Could you check a few things on this model? Use its own coordinates, in mm. A direction names the side the tool comes from. Coordinates: 2 decimals unless noted, no trailing zeros. Loops run counter-clockwise (first coordinate to the right, second up) from the corner with the lowest first, then second, coordinate; pieces in that order, holes last. Notation, with made-up numbers: (24.5, -39) - (52.5, -39) arc R27 ccw to (52.5, -21) - close; hole circle Ø5 at (-20, -38.5). An arc over 180 degrees is marked (long way). Use CSV: the item, a comma, the result in double quotes.
from build123d import *

# Parameters (mm, degrees)
SKETCH1_R               = 27.5
BOSS_EXTRUDE1_DEPTH     = 8
SKETCH2_R               = 26.25
BOSS_EXTRUDE2_DEPTH     = 11
BOSS_EXTRUDE3_DEPTH     = 8
SKETCH4_R               = 5
CUT_EXTRUDE1_DEPTH      = 54.872534746
MIRROR2_OUTLINE_R       = 5
MIRROR2_DEPTH           = 8
SKETCH6_R               = 15
BOSS_EXTRUDE4_DEPTH     = 7
CUT_EXTRUDE2_DEPTH      = 57.055775795
CUT_EXTRUDE2_DEPTH_BACK = 57.055775795
SKETCH5_R               = 10


# Read off the part's stored shape, not the designer's step: Mirror2
with BuildPart() as part:
    # Sketch1 → Boss-Extrude1 (new body)
    with BuildSketch(Plane(origin=(0, 0, 0), x_dir=(1, 0, 0), z_dir=(0, 1, 0))):
        with Locations(Location((0, 0, 0), (0, 0, 270))):
            Circle(SKETCH1_R)
    extrude(amount=BOSS_EXTRUDE1_DEPTH)

    # Sketch2 → Boss-Extrude2 (add)
    with BuildSketch(Plane(origin=(0, 8, 0), x_dir=(1, 0, 0), z_dir=(0, 1, 0))):
        with Locations(Location((0, 0, 0), (0, 0, 270))):
            Circle(SKETCH2_R)
    extrude(amount=BOSS_EXTRUDE2_DEPTH)

    # Sketch3 → Boss-Extrude3 (add)
    with BuildSketch(Plane(origin=(0, 0, 0), x_dir=(1, 0, 0), z_dir=(0, 1, 0))):
        Polygon((20.794342335, 16.0205439), (44.474731406, 6.832149094), (45, 0), (20.794342335, 0), align=None)
    boss_extrude3 = extrude(amount=BOSS_EXTRUDE3_DEPTH)

    # Mirror1: Boss-Extrude3 across plane
    add(boss_extrude3.mirror(Plane.XY))

    # Sketch4 → Cut-Extrude1 (cut, through all)
    with BuildSketch(Plane(origin=(0, 8, 0), x_dir=(1, 0, 0), z_dir=(0, 1, 0))):
        with Locations(Location((35.5, 0, 0), (0, 0, 270))):
            Circle(SKETCH4_R)
    extrude(amount=-CUT_EXTRUDE1_DEPTH, mode=Mode.SUBTRACT)

    # Mirror2 outline → Mirror2 (add)
    with BuildSketch(Plane(origin=(0, 0, 0), x_dir=(1, 0, 0), z_dir=(0, 1, 0))):
        with BuildLine():
            ThreePointArc((-22.9203732, -15.195607667), (-27.5, 0), (-22.9203732, 15.195607667))
            Line((-22.9203732, 15.195607667), (-44.474731406, 6.832149094))
            Line((-44.474731406, 6.832149094), (-45, 0))
            Line((-45, 0), (-44.474731406, -6.832149094))
            Line((-44.474731406, -6.832149094), (-22.9203732, -15.195607667))
        make_face()
        with Locations((-35.5, 0)):
            Circle(MIRROR2_OUTLINE_R, mode=Mode.SUBTRACT)
    extrude(amount=MIRROR2_DEPTH)

    # Sketch6 → Boss-Extrude4 (add)
    with BuildSketch(Plane(origin=(0, 19, 0), x_dir=(1, 0, 0), z_dir=(0, 1, 0))):
        with Locations(Location((0, 0, 0), (0, 0, 270))):
            Circle(SKETCH6_R)
    extrude(amount=BOSS_EXTRUDE4_DEPTH)

    # Sketch5 → Cut-Extrude2 (cut, two sides: drawn at the far end of the back side and taken through both)
    with BuildSketch(Plane(origin=(0, 19, 0), x_dir=(1, 0, 0), z_dir=(0, 1, 0)).offset(-CUT_EXTRUDE2_DEPTH_BACK)):
        with Locations(Location((0, 0, 0), (0, 0, 270))):
            Circle(SKETCH5_R)
    extrude(amount=CUT_EXTRUDE2_DEPTH + CUT_EXTRUDE2_DEPTH_BACK, mode=Mode.SUBTRACT)


solid = part.part
(1) Suppose I cut it at B-B (y = 2.5). Write out the boundary of the cut face in (x, z), plus the area to 3 significant figures.
Computed:
outline,"(-45, 0) - (-44.47, -6.83) - (-22.92, -15.2) arc R27.5 ccw to (22.92, -15.2) - (44.47, -6.83) - (45, 0) - (44.47, 6.83) - (22.92, 15.2) arc R27.5 ccw to (-22.92, 15.2) - (-44.47, 6.83) - close; hole circle Ø10 at (-35.5, 0); hole circle Ø20 at (0, 0); hole circle Ø10 at (35.5, 0)"
area,"2,670 mm²"
(2) Suppose I cut it at A-A (x = 0). Write out the boundary of the cut face in (y, z), plus the area to 4 significant figures.
Computed:
outline,"(0, -27.5) - (8, -27.5) - (8, -26.25) - (19, -26.25) - (19, -15) - (26, -15) - (26, -10) - (0, -10) - close; (0, 10) - (26, 10) - (26, 15) - (19, 15) - (19, 26.25) - (8, 26.25) - (8, 27.5) - (0, 27.5) - close"
area,"707.5 mm²"
(3) Suppose I cut it at D-D (y = 16.75). Write out the boundary of the cut face in (x, z).
Computed:
outline,"circle Ø52.5 at (0, 0); hole circle Ø20 at (0, 0)"
(4) Will these pins go through, and if not, where does the flat tip stop? pin 1 (1.5 mm diameter, centred on y = 9, z = 0, fed in from -X); pin 2 (2 mm diameter, centred on x = -29.5, y = 6, fed in from +Z); pin 3 (6 mm diameter, centred on y = 16, z = 16, fed in from -X); pin 4 (3 mm diameter, centred on x = 24, y = 21.5, fed in from +Z).
Computed:
pin 1,"stops at x = -26.25"
pin 2,"stops at z = 13.03"
pin 3,"stops at x = -22.8"
pin 4,"passes through"
(5) Thinking about a two-plate mould opening in Z: for faces 3 (the face through (0.379, 3.944, -27.497)), 4 (the face through (33.55, 3.94, 11.07)), 5 (the face through (40.457, 4.056, -0.651)), which applies, +Z half, -Z half, draft (parallel to the pull), parting line (faces both ways), or undercut?
Computed:
face 3,"-Z half"
face 4,"+Z half"
face 5,"undercut"
(6) Suppose I cut it at C-C (z = -11.5). Write out the boundary of the cut face in (x, y).
Computed:
outline,"(-32.44, 0) - (32.44, 0) - (32.44, 8) - (23.6, 8) - (23.6, 19) - (9.63, 19) - (9.63, 26) - (-9.63, 26) - (-9.63, 19) - (-23.6, 19) - (-23.6, 8) - (-32.44, 8) - close"
(7) Which directions (+Z, -Z, +X, -X, +Y, -Y) give clear straight access to the entire face, cutting with the end or side of a thin tool? Please do faces 1 (the face through (-0.379, 3.944, 27.497)), 2 (the face through (8, 13, 25)).
Computed:
face 1,"+Z, +Y, -Y"
face 2,"+Y"
(8) Please list where these lines run through material, in increasing order: line 1 (X direction, y = 1.75, z = 0); line 2 (X direction, y = 11, z = 0); line 3 (X direction, y = 7.5, z = -1).
Computed:
line 1,"x = -45 to -40.5, -30.5 to -10, 10 to 30.5, 40.5 to 45"
line 2,"x = -26.25 to -10, 10 to 26.25"
line 3,"x = -44.92 to -40.4, -30.6 to -9.95, 9.95 to 30.6, 40.4 to 44.92"
